```python
from build123d import *

# Parameters (mm, degrees)
SKETCH_1_R          = 2
EXTRUDE_1_DEPTH     = 40
SKETCH_2_R          = 2.1
EXTRUDE_2_DEPTH     = 1.2
CHAMFER_1_SIZE      = 0.2
SKETCH_3_W          = 0.8
SKETCH_3_H          = 4.5
CUT_EXTRUDE_1_DEPTH = 5.5


# Read off the part's stored shape, not the designer's step: 镜向1
with BuildPart() as part:
    # 草图1 → 凸台-拉伸1 (new body)
    with BuildSketch(Plane.XY):
        Circle(SKETCH_1_R)
    extrude(amount=EXTRUDE_1_DEPTH)

    # 草图2 → 凸台-拉伸2 (add)
    with BuildSketch(Plane.XY.offset(40)):
        Circle(SKETCH_2_R)
    extrude(amount=-EXTRUDE_2_DEPTH)

    # 倒角1
    chamfer_1_edges = [part.edges().sort_by_distance(p)[0] for p in [
        (-2.1, 0, 40),
    ]]
    chamfer(chamfer_1_edges, length=CHAMFER_1_SIZE)

    # 草图3 → 切除-拉伸1 (cut)
    with BuildSketch(Plane.XY.offset(40)):
        Rectangle(SKETCH_3_W, SKETCH_3_H)
    extrude(amount=-CUT_EXTRUDE_1_DEPTH, mode=Mode.SUBTRACT)

    # 镜向1: part across plane


with BuildPart() as part_1:
    add(part.part)
    add(part.part.mirror(Plane.XY))


solid = part_1.part
```
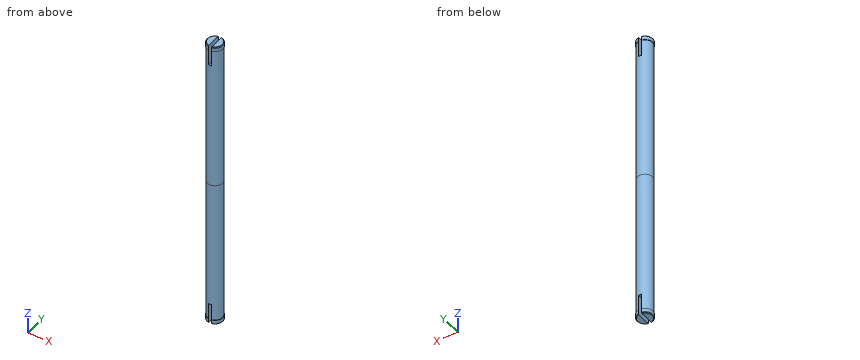
Part model, mm, in its own coordinate system. Coordinates: 2 decimals unless noted, no trailing zeros. Order: outer loops, then holes, each group sorted by start corner. A loop starts at its lowest first (then second) coordinate and runs counter-clockwise, first axis right, second up. Notation, with made-up numbers: (30.25, 7.5) - (78.25, 7.5) arc R14 ccw to (78.25, 17.5) - close; hole circle Ø4 at (14.25, -11.75). An arc over 180 degrees is marked (long way). Return JSON: item names as keys, results as strings. Group by question number.
Item 1: Cut at B-B (z = 22). List the corners of the cut face in (x, y).
Item 2: Cut at A-A (y = 0). List the corners of the cut face in (x, z), plus the area to 3 significant figures.
Item 3: Drill centre lines: probe 1 along X at (y, z) = (0.05, 36.5); probe 2 along X at (y, z) = (0.6, -13); probe 3 along Y at (x, z) = (0.7, 3). Where is each one in solid material? Low to high. Write a range as from..to.
Item 4: Pin check, flat tips, straight feed: pin 1 (1.2 mm diameter, centred on y = 1, z = 36, fed in from -X); pin 2 (2 mm diameter, centred on x = 1.5, z = -16.5, fed in from -Y); pin 3 (0.6 mm diameter, centred on x = 0, y = -1, fed in from -Z). Stop position of each tip, or through.
Check values:
{
 "1": {"outline": "circle Ø4 at (0, 0)"},
 "2": {"outline": "(-2.1, -39.8) - (-1.9, -40) - (-0.4, -40) - (-0.4, -34.5) - (0.4, -34.5) - (0.4, -40) - (1.9, -40) - (2.1, -39.8) - (2.1, -38.8) - (2, -38.8) - (2, 38.8) - (2.1, 38.8) - (2.1, 39.8) - (1.9, 40) - (0.4, 40) - (0.4, 34.5) - (-0.4, 34.5) - (-0.4, 40) - (-1.9, 40) - (-2.1, 39.8) - (-2.1, 38.8) - (-2, 38.8) - (-2, -38.8) - (-2.1, -38.8) - close", "area": "312 mm2"},
 "3": {"probe 1": "x = -2..-0.4, 0.4..2", "probe 2": "x = -1.91..1.91", "probe 3": "y = -1.87..1.87"},
 "4": {"pin 1": "stops at x = -1.96", "pin 2": "stops at y = -1.94", "pin 3": "stops at z = -34.5"}
}
